from build123d import *

# Parameters (mm, degrees)
SKETCH1_W           = 7.25
SKETCH1_H           = 20
SKETCH1_R           = 6
BOSS_EXTRUDE1_DEPTH = 40
SKETCH2_W           = 42
SKETCH2_H           = 22
CUT_EXTRUDE1_DEPTH  = 25
SKETCH3_R           = 2.05
CUT_EXTRUDE2_DEPTH  = 12
SKETCH4_R           = 9.55
CUT_EXTRUDE3_DEPTH  = 5
SKETCH5_R           = 9.55
CUT_EXTRUDE4_DEPTH  = 6
SKETCH7_W           = 6
SKETCH7_H           = 2
SKETCH7_H_2         = 1.8
CUT_EXTRUDE5_DEPTH  = 2.4
BOSS_EXTRUDE3_REACH = 79.413
SKETCH10_R          = 13.5
SKETCH10_R_2        = 10
BOSS_EXTRUDE4_REACH = 54.413
SKETCH11_R          = 10
SKETCH15_R          = 1.85
CUT_EXTRUDE8_DEPTH  = 13.5


with BuildPart() as part:
    # Sketch1 → Boss-Extrude1 (new body)
    with BuildSketch(Plane(origin=(0, 0, 0), x_dir=(1, 0, 0), z_dir=(0, 1, 0))):
        with BuildLine():
            Line((-30.25, -10), (-37.5, -10))
            Line((-37.5, -10), (-37.5, 10))
            Line((-37.5, 10), (-30.25, 10))
            Line((-30.25, 10), (-18.466185313, 10))
            ThreePointArc((-18.466185313, 10), (-13.083157843, 16.426532831), (-5.61521172, 20.235350191))
            Line((-5.61521172, 20.235350191), (-42.5, 10))
            Line((-42.5, 10), (-42.5, -10))
            Line((-42.5, -10), (-5.61521172, -20.235350191))
            ThreePointArc((-5.61521172, -20.235350191), (-13.083157843, -16.426532831), (-18.466185313, -10))
            Line((-18.466185313, -10), (-30.25, -10))
        make_face()
        with Locations((-33.875, 0)):
            Rectangle(SKETCH1_W, SKETCH1_H)
        with BuildLine():
            ThreePointArc((-18.466185313, 10), (-21, 0), (-18.466185313, -10))
            Line((-18.466185313, -10), (9.75, -10))
            Line((9.75, -10), (9.75, 10))
            Line((9.75, 10), (-18.466185313, 10))
        make_face()
        Circle(SKETCH1_R, mode=Mode.SUBTRACT)
        with BuildLine():
            Line((-30.25, 10), (-30.25, -10))
            Line((-30.25, -10), (-18.466185313, -10))
            ThreePointArc((-18.466185313, -10), (-21, 0), (-18.466185313, 10))
            Line((-18.466185313, 10), (-30.25, 10))
        make_face()
        with BuildLine():
            Line((9.75, -10), (-18.466185313, -10))
            ThreePointArc((-18.466185313, -10), (-13.083157843, -16.426532831), (-5.61521172, -20.235350191))
            ThreePointArc((-5.61521172, -20.235350191), (12.709849603, -16.717048874), (21, 0))
            ThreePointArc((21, 0), (12.709849603, 16.717048874), (-5.61521172, 20.235350191))
            ThreePointArc((-5.61521172, 20.235350191), (-13.083157843, 16.426532831), (-18.466185313, 10))
            Line((-18.466185313, 10), (9.75, 10))
            Line((9.75, 10), (17, 10))
            Line((17, 10), (17, -10))
            Line((17, -10), (9.75, -10))
        make_face()
        with Locations((13.375, 0)):
            Rectangle(SKETCH1_W, SKETCH1_H)
    extrude(amount=BOSS_EXTRUDE1_DEPTH)

    # Sketch2 → Cut-Extrude1 (cut)
    with BuildSketch(Plane(origin=(0, 40, 0), x_dir=(1, 0, 0), z_dir=(0, 1, 0))):
        with Locations((-10, 0)):
            Rectangle(SKETCH2_W, SKETCH2_H)
    extrude(amount=-CUT_EXTRUDE1_DEPTH, mode=Mode.SUBTRACT)

    # Sketch3 → Cut-Extrude2 (cut)
    with BuildSketch(Plane(origin=(0, 40, 0), x_dir=(1, 0, 0), z_dir=(0, 1, 0))):
        with Locations((14.75, 5)):
            Circle(SKETCH3_R)
        with Locations((14.75, -5)):
            Circle(SKETCH3_R)
        with Locations((-34.75, 5)):
            Circle(SKETCH3_R)
        with Locations((-34.75, -5)):
            Circle(SKETCH3_R)
    extrude(amount=-CUT_EXTRUDE2_DEPTH, mode=Mode.SUBTRACT)

    # Sketch4 → Cut-Extrude3 (cut)
    with BuildSketch(Plane(origin=(0, 15, 0), x_dir=(1, 0, 0), z_dir=(0, 1, 0))):
        Circle(SKETCH4_R)
    extrude(amount=-CUT_EXTRUDE3_DEPTH, mode=Mode.SUBTRACT)

    # Sketch5 → Cut-Extrude4 (cut)
    with BuildSketch(Plane.XZ):
        Circle(SKETCH5_R)
    extrude(amount=-CUT_EXTRUDE4_DEPTH, mode=Mode.SUBTRACT)

    # Sketch7 → Cut-Extrude5 (cut)
    with BuildSketch(Plane(origin=(0, 40, 0), x_dir=(1, 0, 0), z_dir=(0, 1, 0))):
        with Locations((-34, 0)):
            Rectangle(SKETCH7_W, SKETCH7_H)
        with Locations((14, 0)):
            Rectangle(SKETCH7_W, SKETCH7_H_2)
    extrude(amount=-CUT_EXTRUDE5_DEPTH, mode=Mode.SUBTRACT)

    # Sketch10 → Boss-Extrude3 (add, up to next)
    with BuildSketch(Plane(origin=(-14.44792881, 9.795327955, -48.752531942), x_dir=(-0.168490085, 0.955554754, 0.241921896), z_dir=(0.279007999, -0.189160321, 0.941473796)), mode=Mode.PRIVATE) as boss_extrude3_sk1:
        with Locations((15.161828301, -3.96392858)):
            Circle(SKETCH10_R)
        with Locations((15.161828301, -3.96392858)):
            Circle(SKETCH10_R_2, mode=Mode.SUBTRACT)
    boss_extrude3_tool1 = extrude(boss_extrude3_sk1.sketch, amount=BOSS_EXTRUDE3_REACH, mode=Mode.PRIVATE) - part.part
    add(boss_extrude3_tool1.solids().sort_by_distance((-11.044801, 12.644515, -49.1886))[0])

    # Sketch11 → Boss-Extrude4 (add, up to next)
    with BuildSketch(Plane(origin=(-7.472728833, 5.066319927, -25.215687031), x_dir=(-0.960288778, -0.054959762, 0.273541383), z_dir=(-0.279007999, 0.189160321, -0.941473796)), mode=Mode.PRIVATE) as boss_extrude4_sk1:
        with Locations((-1.242176115, 15.622124238)):
            Circle(SKETCH11_R)
    boss_extrude4_tool1 = extrude(boss_extrude4_sk1.sketch, amount=-BOSS_EXTRUDE4_REACH, mode=Mode.PRIVATE) - part.part
    add(boss_extrude4_tool1.solids().sort_by_distance((-6.279881, 20.450629, -22.478185))[0])

    # Sketch15 → Cut-Extrude8 (cut, symmetric)
    with BuildSketch(Plane(origin=(1.192847783, 0.068269704, -0.339786572), x_dir=(-0.279007999, 0.189160321, -0.941473796), z_dir=(-0.960288778, -0.054959762, 0.273541383))):
        with Locations((39.283206422, -15.622124238)):
            Circle(SKETCH15_R)
    extrude(amount=CUT_EXTRUDE8_DEPTH, both=True, mode=Mode.SUBTRACT)


solid = part.part
The listing builds one solid part. Answer for the finished solid, in the listing's coordinates (mm). A direction names the side the tool comes from. Give positions to 0.01 mm unless a question says otherwise; leave off trailing zeros. Loops run counter-clockwise (first coordinate to the right, second up) from the corner with the lowest first, then second, coordinate; pieces in that order, holes last.
Item 1: Find the intervals of material crossed by line 1 along Z through (x, y) = (-34.75, 35); line 2 along Y through (x, z) = (-16, 7.5); line 3 along X through (y, z) = (35.5, 5), in increasing order.
Derived:
line 1: z = -12.15 to -7.05, -2.95 to 2.95, 7.05 to 12.15
line 2: y = 0 to 15
line 3: x = -42.5 to -36.8, -32.7 to -31, 11 to 12.7, 16.8 to 20.4
Item 2: A cutting plane is placed at D-D (z = 13.5). Give the vertices of the cut face in (x, y), then the cut area to 3 significant figures.
Derived:
outline: (-29.89, 0) - (16.09, 0) - (16.09, 40) - (-29.89, 40) - close
area: 1,840 mm2
Item 3: Determine the mould class of faces 1 (the flat face through (-27.9, 19.72, -14.05)), 2 (the cylindrical face through (-0.169, 14.417, -38.674)), 3 (the cylindrical face through (-21.27, 20.83, -32.29)), 4 (the cylindrical face through (1.818, 24.281, -35.826)) for opening direction Y: +Y half, -Y half, draft (parallel to the pull), parting line (faces both ways), or undercut.
Derived:
face 1: draft
face 2: parting line
face 3: undercut
face 4: undercut
Item 4: A tool of negligible diameter and unlimited length cuts with its end or side. For faces 5 (the flat face through (14, 37.6, 0)), 6 (the cylindrical face through (-18.694, 26.079, -31.132)), from which of +Z, -Z, +X, -X, +Y, -Y can it reach the whole face along a straight path? Write none if from no direction.
Derived:
face 5: +Y
face 6: none
Item 5: A cutting plane is placed at B-B (x = -28.5). Give the vertices of the cut face in (y, z).
Derived:
outline: (0, -13.88) - (40, -13.88) - (40, -11) - (15, -11) - (15, 11) - (40, 11) - (40, 13.88) - (0, 13.88) - close
Item 6: Each of these flat-tipped pins is pushed along its axis until it touches: pin 1 Ø5 at (y, z) = (13.5, -14.5) entering from +X; pin 2 Ø0.9 at (x, z) = (13, 0) entering from +Y; pin 3 Ø3 at (y, z) = (17.5, -30.5) entering from +X; pin 4 Ø11.5 at (x, z) = (0, 0) entering from +Y. Where does it stop, or does it pass through?
Derived:
pin 1: stops at x = 17.23
pin 2: stops at y = 37.6
pin 3: stops at x = 5.51
pin 4: passes through
Item 7: A cutting plane is placed at C-C (x = 14.75). Give the vertices of the cut face in (y, z).
Derived:
outline: (0, -14.95) - (40, -14.95) - (40, -7.05) - (28, -7.05) - (28, -2.95) - (40, -2.95) - (40, -0.9) - (37.6, -0.9) - (37.6, 0.9) - (40, 0.9) - (40, 2.95) - (28, 2.95) - (28, 7.05) - (40, 7.05) - (40, 14.95) - (0, 14.95) - close
Item 8: A cutting plane is placed at A-A (z = -5). Give the vertices of the cut face in (x, y), then the cut area to 3 significant figures.
Derived:
outline: (-42.5, 0) - (-8.14, 0) - (-8.14, 6) - (-3.32, 6) - (-3.32, 10) - (-8.14, 10) - (-8.14, 15) - (-31, 15) - (-31, 40) - (-32.7, 40) - (-32.7, 28) - (-36.8, 28) - (-36.8, 40) - (-42.5, 40) - close; (3.32, 6) - (8.14, 6) - (8.14, 0) - (20.4, 0) - (20.4, 40) - (16.8, 40) - (16.8, 28) - (12.7, 28) - (12.7, 40) - (11, 40) - (11, 15) - (8.14, 15) - (8.14, 10) - (3.32, 10) - close
area: 1,160 mm2
